For this review, take the finished solid that the model builds, in its own axes (mm). Give positions to 0.01 mm unless a question says otherwise; leave off trailing zeros. Write each loop counter-clockwise with the first axis right and the second up, starting at its lowest first coordinate (ties: lowest second). Pieces come first, ordered by that corner, then holes. Notation, with made-up numbers: M -13,6 L 38,6 A16 cw 38,30 Z; hole C 68.25,27.5 d2. An arc over 180 degrees is marked long. One line per item, written item: value. Start each with the question number.
Item 1: To check wall thickness, follow probe 1 along X at (y, z) = (2.8, 45); probe 2 along X at (y, z) = (4.3, 48); probe 3 along Z at (x, y) = (-32.5, 1.3). State the ranges of each line that lie inside material, in increasing order.
Item 2: Consider section D-D, the plane z = 45. Write out the cut boundary in (x, y).
Item 3: Consider section B-B, the plane x = -20.5. Write out the cut boundary in (y, z).
Item 4: Consider section C-C, the plane z = -30. Write out the cut boundary in (x, y), and give its area (3 significant figures).
Item 5: Consider section A-A, the plane y = 1.3. Write out the cut boundary in (x, z).
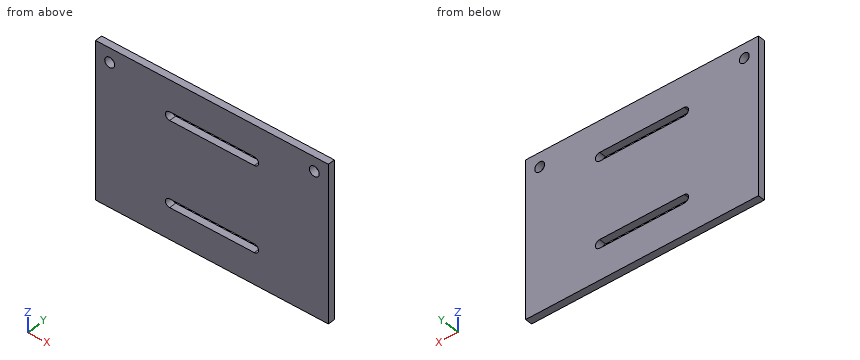
```python
from build123d import *

# Parameters (mm, degrees)
SKETCH1_W           = 165
SKETCH1_H           = 110
SKETCH1_R           = 3.5
BOSS_EXTRUDE1_DEPTH = 5


with BuildPart() as part:
    # Sketch1 → Boss-Extrude1 (new body)
    with BuildSketch(Plane(origin=(0, 0, 0), x_dir=(1, 0, 0), z_dir=(0, 1, 0))):
        Rectangle(SKETCH1_W, SKETCH1_H)
        with Locations(Location((72.5, -45, 0), (0, 0, 270))):
            Circle(SKETCH1_R, mode=Mode.SUBTRACT)
        with Locations(Location((-72.5, -45, 0), (0, 0, 270))):
            Circle(SKETCH1_R, mode=Mode.SUBTRACT)
        with BuildLine():
            Line((30, -33), (-30, -33))
            ThreePointArc((-30, -33), (-33, -30), (-30, -27))
            Line((-30, -27), (30, -27))
            ThreePointArc((30, -27), (33, -30), (30, -33))
        make_face(mode=Mode.SUBTRACT)
        with BuildLine():
            Line((30, 27), (-30, 27))
            ThreePointArc((-30, 27), (-33, 30), (-30, 33))
            Line((-30, 33), (30, 33))
            ThreePointArc((30, 33), (33, 30), (30, 27))
        make_face(mode=Mode.SUBTRACT)
    extrude(amount=BOSS_EXTRUDE1_DEPTH)


solid = part.part
```
Model answer:
1. probe 1: x = -82.5 to -76, -69 to 69, 76 to 82.5
1. probe 2: x = -82.5 to -74.3, -70.7 to 70.7, 74.3 to 82.5
1. probe 3: z = -55 to -31.66, -28.34 to 28.34, 31.66 to 55
2. outline: M -82.5,0 L -76,0 L -76,5 L -82.5,5 Z; M -69,0 L 69,0 L 69,5 L -69,5 Z; M 76,0 L 82.5,0 L 82.5,5 L 76,5 Z
3. outline: M 0,-55 L 5,-55 L 5,-33 L 0,-33 Z; M 0,-27 L 5,-27 L 5,27 L 0,27 Z; M 0,33 L 5,33 L 5,55 L 0,55 Z
4. outline: M -82.5,0 L -33,0 L -33,5 L -82.5,5 Z; M 33,0 L 82.5,0 L 82.5,5 L 33,5 Z
4. area: 495 mm2
5. outline: M -82.5,-55 L 82.5,-55 L 82.5,55 L -82.5,55 Z; hole C -72.5,45 d7; hole M -30,-33 L 30,-33 A3 ccw 30,-27 L -30,-27 A3 ccw Z; hole M -30,27 L 30,27 A3 ccw 30,33 L -30,33 A3 ccw Z; hole C 72.5,45 d7
